Verification items for the finished model (mm, model axes). A direction names the side the tool comes from. Give positions to 0.01 mm unless a question says otherwise; leave off trailing zeros. Order: outer loops, then holes, each group sorted by start corner. A loop starts at its lowest first (then second) coordinate and runs counter-clockwise, first axis right, second up. Notation, with made-up numbers: M 81.5,65.25 L 94.5,65.25 A7 ccw 94.5,76.25 Z; hole C 54.5,41.25 d11. An arc over 180 degrees is marked long. Answer as a JSON object with one key per item and string values.
Autodesk Inventor part; units mm, degrees
ref_plane "YZ Plane" through (0, 0, 0) normal (1, 0, 0) x (0, 1, 0)
ref_plane "XZ Plane" through (0, 0, 0) normal (0, 1, 0) x (-1, 0, 0)
ref_plane "XY Plane" through (0, 0, 0) normal (0, 0, 1) x (1, 0, 0)
sketch "Sketch1" plane through (0, 0, 0) normal (0, 1, 0) x (-1, 0, 0)
  line L0 (-18, 18) -> (18, 18)
  line L1 (18, 18) -> (18, -18)
  line L2 (18, -18) -> (-18, -18)
  line L3 (-18, -18) -> (-18, 18)
  line L4 (-18, 18) -> (18, -18) construction
  line L5 (18, 18) -> (-18, -18) construction
  circle A0 centre (0, 0) radius 16 construction
  circle A1 centre (15.5, 15.5) radius 1.65
  circle A2 centre (15.5, -15.5) radius 1.65
  circle A3 centre (-15.5, -15.5) radius 1.65
  circle A4 centre (-15.5, 15.5) radius 1.65
  circle A5 centre (15.5, 15.5) radius 2.5 construction
  circle A6 centre (15.5, -15.5) radius 2.5
  circle A7 centre (-15.5, -15.5) radius 2.5
  circle A8 centre (-15.5, 15.5) radius 2.5 construction
  point P0 (0, 0)
  dimension "d0" = 36
  dimension "d1" = 36
  dimension "d2" = 32
  dimension "d3" = 3.3
  dimension "d4" = 3.3
  dimension "d5" = 3.3
  dimension "d6" = 5
  dimension "d7" = 5
  dimension "d8" = 5
  dimension "d9" = 5
  dimension "d10" = 3.3
extrude "Extrusion1" add sketch "Sketch1" along normal blind 7.5
fillet "Fillet1" radius 2.5 4 edges at (18, 3.75, 18) (18, 3.75, -18) (-18, 3.75, -18) (-18, 3.75, 18)
sketch "Sketch2" plane through (0, 7.5, 0) normal (0, 1, 0) x (1, 0, 0)
  circle A0 centre (0, 0) radius 17.6
  dimension "d14" = 35.2
extrude "Extrusion2" cut sketch "Sketch2" against normal blind 1.7
sketch "Sketch3" plane through (0, 5.8, 0) normal (0, 1, 0) x (1, 0, 0)
  circle A0 centre (0, 0) radius 16
  dimension "d17" = 32
extrude "Extrusion3" cut sketch "Sketch3" against normal through all
properties part number "Bearing Block P1" material "Aluminum 6061"
Q1. Release check for a two-part mould opening along Z. For faces 1 (the face through (4, 5.8, 16)), 2 (the face through (17.248, 3.802, 17.287)), 3 (the face through (-17.248, 3.802, -17.287)), 4 (the face through (-3.47, 2.94, 15.62)) record: +Z half, -Z half, draft (parallel to the pull), parting line (faces both ways), or undercut.
Resolved:
{"face 1": "undercut", "face 2": "+Z half", "face 3": "-Z half", "face 4": "undercut"}
Q2. Section check A-A on z = -12. Record the cut outline in (x, y).
Resolved:
{"outline": "M -18,0 L -10.58,0 L -10.58,5.8 L -12.87,5.8 L -12.87,7.5 L -18,7.5 Z; M 10.58,0 L 18,0 L 18,7.5 L 12.87,7.5 L 12.87,5.8 L 10.58,5.8 Z"}
Q3. Material ranges on L1, parallel to Z at x = 0, y = 2.75; L2, parallel to X at y = 6.4, z = 0; L3, parallel to Z at x = 4, y = 5.25, recorded low to high.
Resolved:
{"L1": "z = -18 to -16, 16 to 18", "L2": "x = -18 to -17.6, 17.6 to 18", "L3": "z = -18 to -15.49, 15.49 to 18"}
Q4. Tool access check on faces 5 (the face through (16.787, 6.662, -5.287)), 6 (the face through (0, 4, 18)). Record the directions out of +Z, -Z, +X, -X, +Y, -Y that give a thin tool (end or side, any length) a straight path to the whole face; none if there is none.
Resolved:
{"face 5": "+Y", "face 6": "+Z, +X, -X, +Y, -Y"}
Q5. Section check C-C on x = 6. Record the cut outline in (y, z).
Resolved:
{"outline": "M 0,-18 L 7.5,-18 L 7.5,-16.55 L 5.8,-16.55 L 5.8,-14.83 L 0,-14.83 Z; M 0,14.83 L 5.8,14.83 L 5.8,16.55 L 7.5,16.55 L 7.5,18 L 0,18 Z"}
Q6. Gauge pin test, flat ends, axial feed: pin 1 Ø4 at (x, z) = (-15.5, -15.5) entering from -Y; pin 2 Ø3 at (x, z) = (15.5, -15.5) entering from +Y. Record the tip position at first contact, or that the pin passes through.
Resolved:
{"pin 1": "stops at y = 0", "pin 2": "passes through"}
Q7. Section check B-B on y = 3.5. Record the cut outline in (x, z).
Resolved:
{"outline": "M -18,-15.5 A2.5 ccw -15.5,-18 L 15.5,-18 A2.5 ccw 18,-15.5 L 18,15.5 A2.5 ccw 15.5,18 L -15.5,18 A2.5 ccw -18,15.5 Z; hole C -15.5,-15.5 d3.3; hole C -15.5,15.5 d3.3; hole C 0,0 d32; hole C 15.5,-15.5 d3.3; hole C 15.5,15.5 d3.3"}
